```python
from build123d import *

# Parameters (mm, degrees)
SKETCH1_R           = 2.4892
BOSS_EXTRUDE1_DEPTH = 3.175


with BuildPart() as part:
    # Sketch1 → Boss-Extrude1 (new body)
    with BuildSketch(Plane(origin=(0, 0, 0), x_dir=(1, 0, 0), z_dir=(0, 1, 0))):
        with BuildLine():
            Line((-32.037640644, 123.979709158), (-111.412640644, 123.979709158))
            ThreePointArc((-111.412640644, 123.979709158), (-115.902768704, 122.119837219), (-117.762640644, 117.629709158))
            Line((-117.762640644, 117.629709158), (-117.762640644, 27.967709158))
            ThreePointArc((-117.762640644, 27.967709158), (-115.902768704, 23.477581098), (-111.412640644, 21.617709158))
            Line((-111.412640644, 21.617709158), (-47.412584086, 21.687857346))
            Line((-47.412584086, 21.687857346), (-47.412584086, 15.168903158))
            ThreePointArc((-47.412584086, 15.168903158), (-49.243516418, 10.748641491), (-53.663778086, 8.917709158))
            Line((-53.663778086, 8.917709158), (-98.720178026, 8.917709158))
            ThreePointArc((-98.720178026, 8.917709158), (-123.447337141, 7.816048009), (-147.978557367, 4.519794164))
            Line((-147.978557367, 4.519794164), (-154.737719104, 3.303145051))
            ThreePointArc((-154.737719104, 3.303145051), (-162.112204751, 8.427787619), (-156.987562183, 15.802273266))
            Line((-156.987562183, 15.802273266), (-156.510910789, 15.888070517))
            ThreePointArc((-156.510910789, 15.888070517), (-137.832620256, 26.738584362), (-130.462640644, 47.043647486))
            Line((-130.462640644, 47.043647486), (-130.462640644, 134.142309925))
            Line((-130.462640644, 134.142309925), (-122.659506644, 141.945443925))
            Line((-122.659506644, 141.945443925), (58.584225356, 141.945443925))
            Line((58.584225356, 141.945443925), (66.387359356, 134.142309925))
            Line((66.387359356, 134.142309925), (66.387359356, 47.043647486))
            ThreePointArc((66.387359356, 47.043647486), (73.757338969, 26.738584362), (92.435629502, 15.888070517))
            Line((92.435629502, 15.888070517), (92.912280896, 15.802273266))
            ThreePointArc((92.912280896, 15.802273266), (98.036923464, 8.427787619), (90.662437817, 3.303145051))
            Line((90.662437817, 3.303145051), (83.90327608, 4.519794164))
            ThreePointArc((83.90327608, 4.519794164), (69.690534676, 6.700322348), (55.384073682, 8.143199745))
            ThreePointArc((55.384073682, 8.143199745), (49.05429115, 11.190619944), (46.487475356, 17.730067432))
            Line((46.487475356, 17.730067432), (46.487475356, 21.600342717))
            ThreePointArc((46.487475356, 21.600342717), (46.487422167, 21.617708833), (46.487262601, 21.635074297))
            Line((46.487262601, 21.635074297), (46.485354971, 21.790775541))
            Line((46.485354971, 21.790775541), (48.820465356, 21.793334972))
            ThreePointArc((48.820465356, 21.793334972), (52.324353596, 24.036756545), (53.687359356, 27.967709158))
            Line((53.687359356, 27.967709158), (53.687359356, 117.629709158))
            ThreePointArc((53.687359356, 117.629709158), (51.827487417, 122.119837219), (47.337359356, 123.979709158))
            Line((47.337359356, 123.979709158), (-32.037640644, 123.979709158))
        make_face()
        with Locations((60.037359356, 119.407709158)):
            Circle(SKETCH1_R, mode=Mode.SUBTRACT)
        with Locations((-52.542234775, 15.267709158)):
            Circle(SKETCH1_R, mode=Mode.SUBTRACT)
        with Locations((-78.392640644, 15.267709158)):
            Circle(SKETCH1_R, mode=Mode.SUBTRACT)
        with Locations((-10.796890644, 133.504709158)):
            Circle(SKETCH1_R, mode=Mode.SUBTRACT)
        with Locations((31.684609356, 133.504709158)):
            Circle(SKETCH1_R, mode=Mode.SUBTRACT)
        with Locations((91.787359356, 9.552709158)):
            Circle(SKETCH1_R, mode=Mode.SUBTRACT)
        with Locations((-53.278390644, 133.504709158)):
            Circle(SKETCH1_R, mode=Mode.SUBTRACT)
        with Locations((-95.759890644, 133.504709158)):
            Circle(SKETCH1_R, mode=Mode.SUBTRACT)
        with Locations((-124.112640644, 15.267709158)):
            Circle(SKETCH1_R, mode=Mode.SUBTRACT)
        with Locations((-155.862640644, 9.552709158)):
            Circle(SKETCH1_R, mode=Mode.SUBTRACT)
        with Locations((-124.112640644, 119.407709158)):
            Circle(SKETCH1_R, mode=Mode.SUBTRACT)
        with Locations((60.037359356, 15.267709158)):
            Circle(SKETCH1_R, mode=Mode.SUBTRACT)
    extrude(amount=BOSS_EXTRUDE1_DEPTH)


solid = part.part
```
Geometry check sheet. Reference: the model listing, model coordinates, mm. A direction names the side the tool comes from. Round coordinates to 2 decimals unless told otherwise and drop trailing zeros. Loops run counter-clockwise (first coordinate to the right, second up) from the corner with the lowest first, then second, coordinate; pieces in that order, holes last. Notation, with made-up numbers: M 58,27 L 71,27 A35 cw 71,59 Z; hole C 74,68 d7. An arc over 180 degrees is marked long. Return JSON: item names as keys, results as strings. Group by question number.
(1) Section check B-B, the plane x = -73. Enter the section's corners in (y, z) (3 decimals).
(2) Set-up check for faces 5 (the face through (-49.195, 1.565, -10.798)), 6 (the face through (-115.952, 1.565, -23.527)), 7 (the face through (-31.4, 3.175, -124.3)): record each of +Z, -Z, +X, -X, +Y, -Y from which the full face is reachable in a straight line by a thin tool's end or side.
(3) Go/stop test with flat-tipped pins: pin 1 (4.5 mm diameter, centred on x = 31.68, z = -133.5, fed in from -Y); pin 2 (1.6 mm diameter, centred on y = 2, z = -93, fed in from -X); pin 3 (1 mm diameter, centred on y = 1.5, z = -19.5, fed in from -X); pin 4 (1.6 mm diameter, centred on y = 2.5, z = -94, fed in from +X). Record where each tip stops, or that it passes through.
(4) Mould release check, pull along Z, two halves, no side actions. Record for faces 1 (the face through (89.3, 1.57, -9.66)), 2 (the face through (-162.086, 1.565, -8.291)), 3 (the face through (-138.032, 1.565, -26.503)), 4 (the face through (-55.03, 1.57, -15.38)): pulls with the +Z half, pulls with the -Z half, needs draft (parallel to the pull), parting line crosses it, or undercut.
(5) Section check C-C, the plane y = 1.65. Give the number of separate pieces and of enclosed holes in the cut face, and give its area (3 significant figures).
(6) Section check A-A, the plane z = -111. Enter the section's corners in (x, y) (3 decimals).
(7) Scan lines: line 1 along X through (y, z) = (1.15, -71); line 2 along X through (y, z) = (1.5, -13); line 3 along Z through (x, y) = (-79, 1.95). Record each from-to range of solid material in increasing order. Write a range as [from, to].
(8) Section check D-D, the plane x = -39.5. Enter the section's corners in (y, z) (3 decimals), and give its area (3 significant figures).
Data:
{
 "1": {"outline": "M 0,-141.945 L 3.175,-141.945 L 3.175,-123.98 L 0,-123.98 Z; M 0,-21.66 L 3.175,-21.66 L 3.175,-8.918 L 0,-8.918 Z"},
 "2": {"face 5": "+Z, +Y, -Y", "face 6": "+Y, -Y", "face 7": "+Z, -Z, +X, -X, +Y"},
 "3": {"pin 1": "through", "pin 2": "x = -130.46", "pin 3": "x = -147.43", "pin 4": "x = 66.39"},
 "4": {"face 1": "undercut", "face 2": "parting line crosses it", "face 3": "pulls with the -Z half", "face 4": "undercut"},
 "5": {"separate pieces": "1", "enclosed holes": "12", "area": "8,270 mm²"},
 "6": {"outline": "M -130.463,0 L -117.763,0 L -117.763,3.175 L -130.463,3.175 Z; M 53.687,0 L 66.387,0 L 66.387,3.175 L 53.687,3.175 Z"},
 "7": {"line 1": "[-130.46, -117.76], [53.69, 66.39]", "line 2": "[-161.2, -125.14], [-123.09, -79.42], [-77.37, -53.57], [-51.52, -47.8], [47.73, 59.01], [61.06, 97.12]", "line 3": "[-141.95, -123.98], [-21.65, -17.68], [-12.85, -8.92]"},
 "8": {"outline": "M 0,-141.945 L 3.175,-141.945 L 3.175,-123.98 L 0,-123.98 Z", "area": "57.0 mm²"}
}
